```python
from build123d import *

# Parameters (mm, degrees)
EXTRUDE_1_DEPTH     = 8
SKETCH_2_R          = 0.6
CUT_EXTRUDE_1_DEPTH = 14.747727085
HOLE_WIZARD_M3_1_D  = 3.4
FILLET_1_R          = 1


with BuildPart() as part:
    # ｽｹｯﾁ1 → ﾎﾞｽ - 押し出し1 (new body)
    with BuildSketch(Plane.XY):
        Polygon((-5, -6), (5, -6), (5, 6), (2, 6), (2, -4), (-5, -4), align=None)
    extrude(amount=EXTRUDE_1_DEPTH)

    # ｽｹｯﾁ2 → ｶｯﾄ - 押し出し1 (cut, through all)
    with BuildSketch(Plane(origin=(0, -4, 0), x_dir=(1, 0, 0), z_dir=(0, 1, 0))):
        with Locations(Location((-1.11, -4, 0), (0, 0, 180))):
            Circle(SKETCH_2_R)
        with Locations(Location((-3.65, -4, 0), (0, 0, 180))):
            Circle(SKETCH_2_R)
    extrude(amount=-CUT_EXTRUDE_1_DEPTH, mode=Mode.SUBTRACT)

    # M3 すきま穴1 (through all)
    with Locations(Plane.ZY.offset(-2)):
        with Locations((4, 3)):
            Hole(HOLE_WIZARD_M3_1_D / 2)

    # ﾌｨﾚｯﾄ1
    fillet_1_edges = [part.edges().sort_by_distance(p)[0] for p in [
        (2, -4, 4),
    ]]
    fillet(fillet_1_edges, radius=FILLET_1_R)


solid = part.part
```
Input: part model. Units: mm. Frame: model coordinates. A direction names the side the tool comes from. Coordinates: 2 decimals unless noted, no trailing zeros. Loops run counter-clockwise (first coordinate to the right, second up) from the corner with the lowest first, then second, coordinate; pieces in that order, holes last. Notation, with made-up numbers: (-39.75, 85.5) - (-9.75, 85.5) arc R9 ccw to (-9.75, 101.5) - close; hole circle Ø5 at (-32, 41.5). An arc over 180 degrees is marked (long way). Answer in a Markdown table with one row per item.
(1) Mould query, pull axis Z, two halves, no side actions, for faces 1 (the face through (3.521, 4.433, 3.086)), 2 (the face through (-1.032, -4.986, 4.595)), 3 (the face through (2.2, -1.2, 8)), 4 (the face through (4, 6, 4)). Classes: pulls with the +Z half, pulls with the -Z half, needs draft (parallel to the pull), parting line crosses it, or undercut.
Model answer:
| item | result |
|---|---|
| face 1 | undercut |
| face 2 | undercut |
| face 3 | pulls with the +Z half |
| face 4 | needs draft |
(2) Cut plane C-C on z = 2.75. Output: boundary loops of the cut face in (x, y), plus the area to 3 significant figures.
Model answer:
| item | result |
|---|---|
| outline | (-5, -6) - (5, -6) - (5, 1.85) - (2, 1.85) - (2, -3) arc R1 cw to (1, -4) - (-5, -4) - close; (2, 4.15) - (5, 4.15) - (5, 6) - (2, 6) - close |
| area | 43.3 mm² |
(3) Material intervals for L1, parallel to Y at x = 3.15, z = 4; L2, parallel to Z at x = -3.65, y = -4.9; L3, parallel to X at y = 0.75, z = 6, sorted ascending. Write a range as from..to.
Model answer:
| item | result |
|---|---|
| L1 | y = -6..1.3, 4.7..6 |
| L2 | z = 0..3.4, 4.6..8 |
| L3 | x = 2..5 |
(4) Pin query (flat end, axial travel): P1, Ø4, axis at x = -1.5, z = 3.5, coming from the +Y side; P2, Ø2, axis at y = 4, z = 6.5, coming from the -X side. Return the tip coordinate at first contact, or that it passes through.
Model answer:
| item | result |
|---|---|
| P1 | stops at y = -4 |
| P2 | stops at x = 2 |
(5) Cut plane A-A on y = 3. Output: boundary loops of the cut face in (x, z), plus the area to 3 significant figures.
Model answer:
| item | result |
|---|---|
| outline | (2, 0) - (5, 0) - (5, 2.3) - (2, 2.3) - close; (2, 5.7) - (5, 5.7) - (5, 8) - (2, 8) - close |
| area | 13.8 mm² |
(6) Cut plane B-B on x = -3.65. Output: boundary loops of the cut face in (y, z), plus the area to 3 significant figures.
Model answer:
| item | result |
|---|---|
| outline | (-6, 0) - (-4, 0) - (-4, 3.4) - (-6, 3.4) - close; (-6, 4.6) - (-4, 4.6) - (-4, 8) - (-6, 8) - close |
| area | 13.6 mm² |
(7) Cut plane D-D on x = 4.25. Output: boundary loops of the cut face in (y, z).
Model answer:
| item | result |
|---|---|
| outline | (-6, 0) - (6, 0) - (6, 8) - (-6, 8) - close; hole circle Ø3.4 at (3, 4) |
(8) Set-up query: faces 5 (the face through (-2, -4, 4)), 6 (the face through (2.2, -1.2, 0)). Return all of +Z, -Z, +X, -X, +Y, -Y with unobstructed straight access to the full face (end or side cutting, diameter ignored); none if empty.
Model answer:
| item | result |
|---|---|
| face 5 | +Z, -Z, -X, +Y |
| face 6 | -Z, +X, -X, +Y, -Y |
